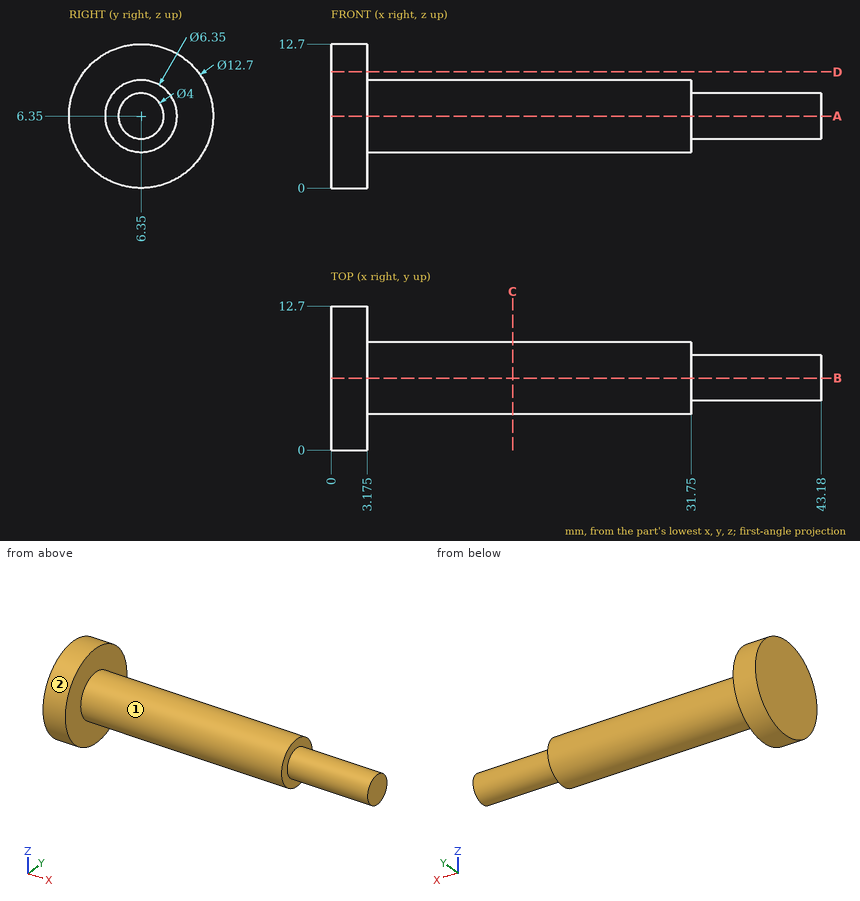
Drawing for the job (mm, zero at the part's lowest x, y, z). A direction names the side the tool comes from. Give positions to 0.01 mm unless a question says otherwise; leave off trailing zeros. Order: outer loops, then holes, each group sorted by start corner. A loop starts at its lowest first (then second) coordinate and runs counter-clockwise, first axis right, second up. Notation, with made-up numbers: M -11.5,80.25 L -7.5,80.25 A30 ccw -7.5,107.25 Z; hole C 82,87.5 d6. An arc over 180 degrees is marked long. Put each result on its own line as item: value.
Item 1: Probe line 1 (X direction, y = 8.5, z = 6.75); line 2 (X direction, y = 4, z = 9.5) (3 decimals); line 3 (Z direction, x = 26.5, y = 6.5). List the from-to ranges inside material, lowest first. Write a range as [from, to].
From the geometry:
line 1: x = [0, 31.75]
line 2: x = [0, 3.175]
line 3: z = [3.18, 9.52]
Item 2: Slice it at D-D, the plane z = 10.25. Write the cut outline in (x, y) (3 decimals).
From the geometry:
outline: M 0,1.339 L 3.175,1.339 L 3.175,11.361 L 0,11.361 Z
Item 3: 3-axis set-ups, long thin cutter, end or side, ignore diameter. For the marked faces 1 and 2: which of +Z, -Z, +X, -X, +Y, -Y reach the whole face in a straight line?
From the geometry:
face 1: +X
face 2: +X, -X
Item 4: Slice it at A-A, the plane z = 6.35. Write the cut outline in (x, y) (3 decimals), plus the area to 3 significant figures.
From the geometry:
outline: M 0,0 L 3.175,0 L 3.175,3.175 L 31.75,3.175 L 31.75,4.35 L 43.18,4.35 L 43.18,8.35 L 31.75,8.35 L 31.75,9.525 L 3.175,9.525 L 3.175,12.7 L 0,12.7 Z
area: 267 mm2
Item 5: Flat gauge pins, fed straight in: pin 1 Ø3 at (x, y) = (29.5, 5.5) entering from -Z (3 decimals); pin 2 Ø6 at (x, z) = (18.5, 10) entering from -Y; pin 3 Ø6 at (x, y) = (15.5, 4) entering from +Z (3 decimals). Where does each tip first touch, or does it go through?
From the geometry:
pin 1: stops at z = 3.175
pin 2: stops at y = 3.24
pin 3: stops at z = 9.525
Item 6: Slice it at C-C, the plane x = 16. Write the cut outline in (y, z) (3 decimals).
From the geometry:
outline: C 6.35,6.35 d6.35
